from build123d import *

# Parameters (mm, degrees)
SKETCH_2_R      = 1.5
EXTRUDE_3_DEPTH = 4
FILLET_1_R      = 3


with BuildPart() as part:
    # 草图2 → 凸台-拉伸3 (new body)
    with BuildSketch(Plane.XY):
        Polygon((-83.375314497, 134.732138716), (-83.375314497, -47.467861284), (-10.875314497, -47.467861284), (-10.875314497, -22.467861284), (-73.375314497, -22.467861284), (-73.375314497, 111.232138716), (54.944685503, 111.232138716), (54.944685503, 134.732138716), align=None)
        with Locations((-59.645314497, -33.737861284)):
            Circle(SKETCH_2_R, mode=Mode.SUBTRACT)
        with Locations((-15.875314497, -37.467861284)):
            Circle(SKETCH_2_R, mode=Mode.SUBTRACT)
        with Locations((-78.375314497, -8.737861284)):
            Circle(SKETCH_2_R, mode=Mode.SUBTRACT)
        with Locations((-80.875314497, 42.532138716)):
            Circle(SKETCH_2_R, mode=Mode.SUBTRACT)
        with Locations((-78.375314497, 93.802138716)):
            Circle(SKETCH_2_R, mode=Mode.SUBTRACT)
        with Locations((-59.645314497, 118.802138716)):
            Circle(SKETCH_2_R, mode=Mode.SUBTRACT)
        with Locations((-30.875314497, 119.732138716)):
            Circle(SKETCH_2_R, mode=Mode.SUBTRACT)
        with Locations((-30.875314497, 129.732138716)):
            Circle(SKETCH_2_R, mode=Mode.SUBTRACT)
        with BuildLine():
            ThreePointArc((25.644685503, 131.232138716), (27.144685503, 129.732138716), (25.644685503, 128.232138716))
            Line((25.644685503, 128.232138716), (18.644685503, 128.232138716))
            ThreePointArc((18.644685503, 128.232138716), (17.144685503, 129.732138716), (18.644685503, 131.232138716))
            Line((18.644685503, 131.232138716), (25.644685503, 131.232138716))
        make_face(mode=Mode.SUBTRACT)
        with BuildLine():
            Line((25.644685503, 118.232138716), (18.644685503, 118.232138716))
            ThreePointArc((18.644685503, 118.232138716), (17.144685503, 119.732138716), (18.644685503, 121.232138716))
            Line((18.644685503, 121.232138716), (25.644685503, 121.232138716))
            ThreePointArc((25.644685503, 121.232138716), (27.144685503, 119.732138716), (25.644685503, 118.232138716))
        make_face(mode=Mode.SUBTRACT)
        with Locations((47.044685503, 129.732138716)):
            Circle(SKETCH_2_R, mode=Mode.SUBTRACT)
        with Locations((47.044685503, 119.732138716)):
            Circle(SKETCH_2_R, mode=Mode.SUBTRACT)
    extrude(amount=EXTRUDE_3_DEPTH)

    # 圆角1
    fillet_1_edges = [part.edges().sort_by_distance(p)[0] for p in [
        (-10.875314497, -22.467861284, 2),
        (-10.875314497, -47.467861284, 2),
        (-83.375314497, -47.467861284, 2),
        (-83.375314497, 134.732138716, 2),
        (54.944685503, 134.732138716, 2),
        (54.944685503, 111.232138716, 2),
    ]]
    fillet(fillet_1_edges, radius=FILLET_1_R)


solid = part.part
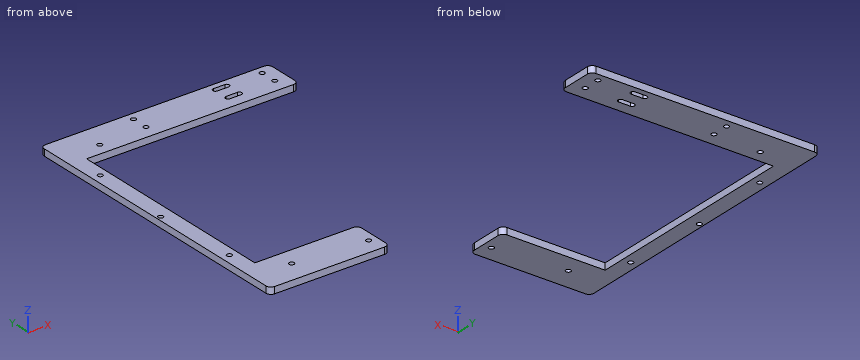
Design review of the part built by this model. Coordinates are the model's own, in mm. Coordinates: 2 decimals unless noted, no trailing zeros. Order: outer loops, then holes, each group sorted by start corner. A loop starts at its lowest first (then second) coordinate and runs counter-clockwise, first axis right, second up. Notation, with made-up numbers: (-36.75, 46) - (2.25, 46) arc R15 cw to (2.25, 50) - close; hole circle Ø5 at (47.5, 59.25). An arc over 180 degrees is marked (long way). Put each result on its own line as item: value.
1) Wall thickness on L1, parallel to Y at x = -28.5, z = 2.7; L2, parallel to Y at x = -17, z = 1.9; L3, parallel to Y at x = -15, z = 0.9: over which ranges is each line inside the solid? List them lowest first. Write a range as from..to.
Response values:
L1: y = -47.47..-22.47, 111.23..134.73
L2: y = -47.47..-38.46, -36.48..-22.47, 111.23..134.73
L3: y = -47.47..-38.69, -36.25..-22.47, 111.23..134.73
2) Take a section at D-D, the plane y = 20. Give the boundary of the cut face in (x, z).
Response values:
outline: (-83.38, 0) - (-73.38, 0) - (-73.38, 4) - (-83.38, 4) - close
3) Insertion check: P1, Ø4, axis at x = -15.88, y = -37.47, coming from the -Z side; P2, Ø1.5, axis at y = 68.5, z = 2.5, coming from the +X side; P3, Ø2, axis at x = 23, z = 2, coming from the -Y side; P4, Ø1.2, axis at y = -36, z = 1.5, coming from the +X side. Each pin has a flat end and moves straight along its axis. Give the tip position at first contact, or say it passes through.
Response values:
P1: stops at z = 0
P2: stops at x = -73.38
P3: stops at y = 111.23
P4: stops at x = -10.88
4) Take a section at B-B, the plane z = 0.8. Count the separate pieces of the cut face and the enclosed holes in it, and give its area (3 significant figures).
Response values:
separate pieces: 1
enclosed holes: 12
area: 6,260 mm²
5) Take a section at A-A, the plane x = -71. Give the boundary of the cut face in (y, z).
Response values:
outline: (-47.47, 0) - (-22.47, 0) - (-22.47, 4) - (-47.47, 4) - close; (111.23, 0) - (134.73, 0) - (134.73, 4) - (111.23, 4) - close
6) Take a section at C-C, the plane x = -1.5. Give the boundary of the cut face in (y, z), and give its area (3 significant figures).
Response values:
outline: (111.23, 0) - (134.73, 0) - (134.73, 4) - (111.23, 4) - close
area: 94.0 mm²
